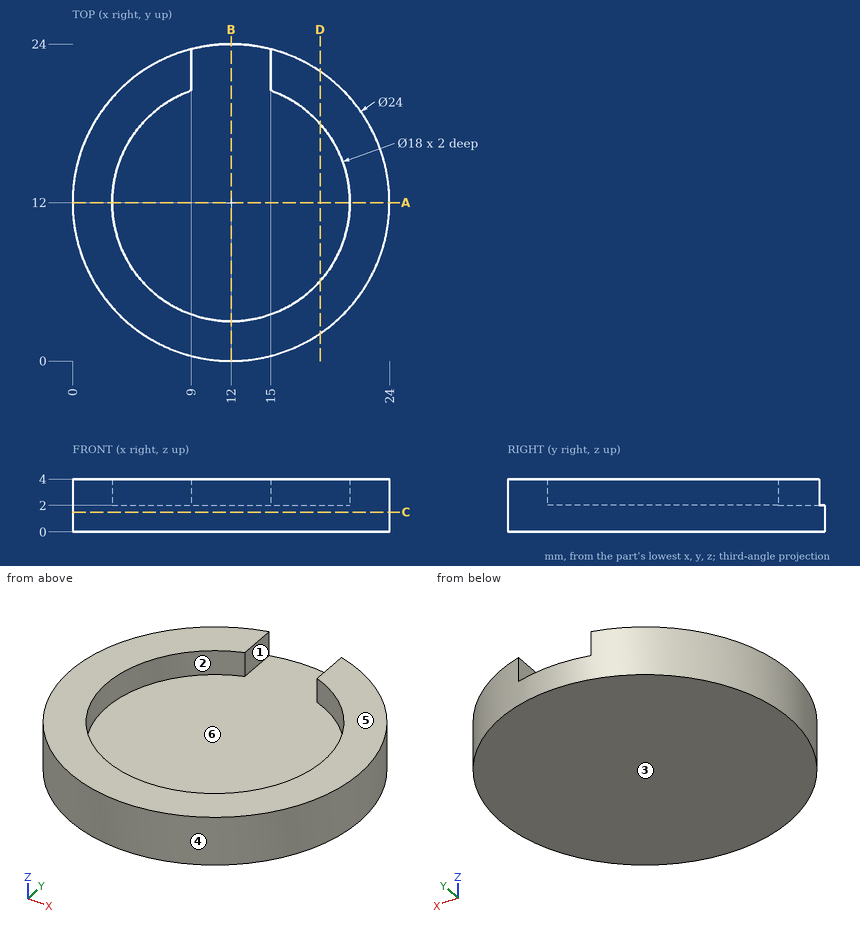
Verification items for this drawing (mm, ordinates from the low corner). A direction names the side the tool comes from. Give positions to 0.01 mm unless a question says otherwise; leave off trailing zeros. Write each loop counter-clockwise with the first axis right and the second up, starting at its lowest first coordinate (ties: lowest second). Pieces come first, ordered by that corner, then holes.
1) Access from +Z, -Z, +X, -X, +Y, -Y to the whole of each face (thin tool, end or side, straight path). Record for the marked faces 1, 2 and 3.
2) Section check D-D, the plane x = 18.75. Record the boundary of the cut face in (y, z), and give its area (3 significant figures).
3) Section check A-A, the plane y = 12. Record the boundary of the cut face in (x, z).
4) Section check B-B, the plane x = 12. Record the boundary of the cut face in (y, z), and give its area (3 significant figures).
5) Release check for a two-part mould opening along X. For the marked faces 4, 5 and 6 record: pulls with the +X half, pulls with the -X half, needs draft (parallel to the pull), parting line crosses it, or undercut.
6) Material ranges on L1, parallel to X at y = 12, z = 3.25; L2, parallel to Z at x = 16.5, y = 5.25; L3, parallel to Y at x = 12, z = 2.65, recorded low to high.
7) Section check C-C, the plane z = 1.5. Record the boundary of the cut face in (x, y), and give its area (3 significant figures).
8) Gauge pin test, flat ends, axial feed: pin 1 (1 mm diameter, centred on y = 22, z = 3.5, fed in from -X); pin 2 (1 mm diameter, centred on y = 22.5, z = 3, fed in from +X); pin 3 (5.5 mm diameter, centred on x = 12.5, y = 17.5, fed in from +Z). Record the tip position at first contact, or that the pin passes through.
Computed:
1. face 1: +Z, +Y
1. face 2: +Z
1. face 3: -Z, +X, -X, +Y, -Y
2. outline: (2.08, 0) - (21.92, 0) - (21.92, 4) - (17.95, 4) - (17.95, 2) - (6.05, 2) - (6.05, 4) - (2.08, 4) - close
2. area: 55.6 mm2
3. outline: (0, 0) - (24, 0) - (24, 4) - (21, 4) - (21, 2) - (3, 2) - (3, 4) - (0, 4) - close
4. outline: (0, 0) - (24, 0) - (24, 2) - (3, 2) - (3, 4) - (0, 4) - close
4. area: 54.0 mm2
5. face 4: parting line crosses it
5. face 5: needs draft
5. face 6: undercut
6. L1: x = 0 to 3, 21 to 24
6. L2: z = 0 to 2
6. L3: y = 0 to 3
7. outline: circle Ø24 at (12, 12)
7. area: 452 mm2
8. pin 1: stops at x = 4.67
8. pin 2: stops at x = 18.63
8. pin 3: stops at z = 2
